Could you check a few things on this model? Use its own coordinates, in mm. Face numbers are marked on the shaded views. A direction names the side the tool comes from. Give positions to 0.01 mm unless a question says otherwise; leave off trailing zeros. Write each loop counter-clockwise with the first axis right and the second up, starting at its lowest first coordinate (ties: lowest second). Pieces come first, ordered by that corner, then holes. Notation, with made-up numbers: (48.5, -0.5) - (100.5, -0.5) arc R29 cw to (100.5, 27.5) - close; hole circle Ø7 at (51.25, -19.5). An arc over 180 degrees is marked (long way). Write item = value, one per line.
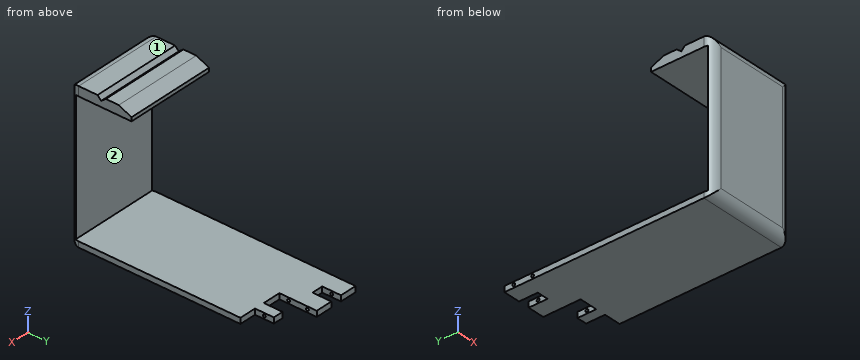
from build123d import *

# Parameters (mm, degrees)
F1_DEPTH      = 3
F3_DEPTH      = 48
F4_T1_DEPTH   = 73.0048285071
F4_T3_DEPTH   = 103.0048285071
F5_R          = 0.75
F6_DEPTH      = 39.001
F7_R          = 0.75
F8_DEPTH      = 9.001
F8_DEPTH_BACK = 39.001


# Not quite as in the source:
# - a fillet or chamfer that OpenCascade refuses, or shapes differently, is made with other operations: its cross-section is extruded or revolved along the edge and cut away or added


with BuildPart() as f1:
    # F0 (on Top) → F1 (new body)
    with BuildSketch(Plane.XY):
        Polygon((-24, 0), (0, 0), (24, 0), (24, 88), (15, 88), (15, 98), (9.6, 98.0832448602), (9.6, 88.0832448602), (0, 88.0832448602), (0, 108), (-9, 108), (-9, 98), (-15, 98), (-15, 108), (-24, 108), align=None)
    extrude(amount=F1_DEPTH)

    # F2 (on face) → F3 (join)
    with BuildSketch(Plane.YZ.offset(24)):
        Polygon((-3.0602848184, 0), (0, 0), (0, 73), (30, 73), (29.9925141591, 74.9999859905), (23.2637450099, 78), (16.367437318, 78), (13.8705000281, 76), (11.9397151816, 78), (-3.0602848184, 78), align=None)
    extrude(amount=-F3_DEPTH)

    # F4: fillet of radius 5 on 6 edges, made by hand

    # F4_s2 → F4_t1 (cut)
    with BuildSketch(Plane.YZ.offset(-36.5024142536)):
        with BuildLine():
            ThreePointArc((-3.0606848184, 72.9990343146), (-1.5958187243, 76.5355339059), (1.9406808671, 78.0004))
            Line((1.9406808671, 78.0004), (1.9406808671, 78.5005365685))
            ThreePointArc((1.9406808671, 78.5005365685), (-0.5598019756, 78.5001365685), (-3.0602848184, 78.5001365685))
            Line((-3.0602848184, 78.5001365685), (-3.5604213869, 78))
            ThreePointArc((-3.5604213869, 78), (-3.5604213869, 75.4995171573), (-3.5608213869, 72.9990343146))
            Line((-3.5608213869, 72.9990343146), (-3.0606848184, 72.9990343146))
        make_face()
        with BuildLine():
            ThreePointArc((1.9406808671, -0.0004), (-1.5958187243, 1.4644660941), (-3.0606848184, 5.0009656854))
            Line((-3.0606848184, 5.0009656854), (-3.5608213869, 5.0009656854))
            ThreePointArc((-3.5608213869, 5.0009656854), (-3.5604213869, 2.5004828427), (-3.5604213869, 0))
            Line((-3.5604213869, 0), (-3.0602848184, -0.5001365685))
            ThreePointArc((-3.0602848184, -0.5001365685), (-0.5598019756, -0.5001365685), (1.9406808671, -0.5005365685))
            Line((1.9406808671, -0.5005365685), (1.9406808671, -0.0004))
        make_face()
    extrude(amount=F4_T1_DEPTH, mode=Mode.SUBTRACT)

    # F4_s4 → F4_t3 (cut)
    with BuildSketch(Plane.XY.offset(-12.5024142536)):
        with BuildLine():
            ThreePointArc((18.9990343146, -3.0606848184), (22.5355339059, -1.5958187243), (24.0004, 1.9406808671))
            Line((24.0004, 1.9406808671), (24.5005365685, 1.9406808671))
            ThreePointArc((24.5005365685, 1.9406808671), (24.5001365685, -0.5598019756), (24.5001365685, -3.0602848184))
            Line((24.5001365685, -3.0602848184), (24, -3.5604213869))
            ThreePointArc((24, -3.5604213869), (21.4995171573, -3.5604213869), (18.9990343146, -3.5608213869))
            Line((18.9990343146, -3.5608213869), (18.9990343146, -3.0606848184))
        make_face()
        with BuildLine():
            ThreePointArc((-18.9990343146, -3.0606848184), (-22.5355339059, -1.5958187243), (-24.0004, 1.9406808671))
            Line((-24.0004, 1.9406808671), (-24.5005365685, 1.9406808671))
            ThreePointArc((-24.5005365685, 1.9406808671), (-24.5001365685, -0.5598019756), (-24.5001365685, -3.0602848184))
            Line((-24.5001365685, -3.0602848184), (-24, -3.5604213869))
            ThreePointArc((-24, -3.5604213869), (-21.4995171573, -3.5604213869), (-18.9990343146, -3.5608213869))
            Line((-18.9990343146, -3.5608213869), (-18.9990343146, -3.0606848184))
        make_face()
    extrude(amount=F4_T3_DEPTH, mode=Mode.SUBTRACT)

    # F5 (on face) → F6 (cut, through all)
    with BuildSketch(Plane.YZ.offset(15)):
        with Locations((93, 1.5)):
            Circle(F5_R)
    extrude(amount=-F6_DEPTH, mode=Mode.SUBTRACT)

    # F7 (on face) → F8 (cut, two sides)
    with BuildSketch(Plane.YZ.offset(-15)) as f8_sk:
        with Locations((103, 1.5)):
            Circle(F7_R)
    extrude(amount=-F8_DEPTH, mode=Mode.SUBTRACT)
    extrude(f8_sk.sketch, amount=F8_DEPTH_BACK, mode=Mode.SUBTRACT)


solid = f1.part
1. If we section it at C-C, the plane z = 35.5: Please give me the cut outline in (x, y), and give its area (3 significant figures).
Filled sheet:
outline = (-23.61, 0) arc R5 ccw to (-19.06, -3.06) - (19.06, -3.06) arc R5 ccw to (23.61, 0) - close
area = 137 mm2
2. For pin 1 (14 mm diameter, centred on x = 8.5, z = 44.5, fed in from +Y); pin 2 (2.5 mm diameter, centred on y = 92, z = 1, fed in from +X); pin 3 (0.9 mm diameter, centred on y = 93, z = 1.5, fed in from -X); pin 4 (3.5 mm diameter, centred on y = 101.5, z = 2, fed in from +X), each with a flat end and sliding along its axis, tell me the tip position at first contact or that it passes through.
Filled sheet:
pin_1 = 0
pin_2 = 15
pin_3 = through
pin_4 = 0
3. If we section it at B-B, the plane y = 5.5: Please give me the cut outline in (x, z), and give its area (3 significant figures).
Filled sheet:
outline = (-24, 0) - (24, 0) - (24, 3) - (-24, 3) - close; (-24, 73) - (24, 73) - (24, 78) - (-24, 78) - close
area = 384 mm2
4. Which directions (+Z, -Z, +X, -X, +Y, -Y) give clear straight access to the entire face, cutting with the end or side of a thin tool? Please do the marked faces 1 and 2.
Filled sheet:
face_1 = +Z, +X, -X, +Y, -Y
face_2 = +X, -X, +Y
5. If we section it at D-D, the plane y = 26: Please give me the cut outline in (x, z), and give its area (3 significant figures).
Filled sheet:
outline = (-24, 0) - (24, 0) - (24, 3) - (-24, 3) - close; (-24, 73) - (24, 73) - (24, 76.78) - (-24, 76.78) - close
area = 325 mm2
6. If we section it at A-A, the plane x = -16.5: Please give me the cut outline in (y, z).
Filled sheet:
outline = (-3.06, 4.94) arc R5 ccw to (1.88, 0) - (108, 0) - (108, 3) - (0, 3) - (0, 73) - (30, 73) - (29.99, 75) - (23.26, 78) - (16.37, 78) - (13.87, 76) - (11.94, 78) - (1.88, 78) arc R5 ccw to (-3.06, 73.06) - close; hole circle Ø1.5 at (93, 1.5); hole circle Ø1.5 at (103, 1.5)
7. I need wall thicknesses on line 1 (Z direction, x = 11.6, y = 93); line 2 (Z direction, x = -9, y = 75); line 3 (Z direction, x = 15.5, y = 25.5). Which ranges of each line are inside material? Lowest first, please.
Filled sheet:
line_1 = 0 to 0.75, 2.25 to 3
line_2 = 0 to 3
line_3 = 0 to 3, 73 to 77
